Here's how the part is built. I have some questions about the finished solid (model axes, mm). Coordinates: 2 decimals unless noted, no trailing zeros. Answer as a JSON object with one key per item and string values. Group by question number.
Q1. I'm going to push flat-ended pins straight in: pin 1 (1.5 mm diameter, centred on x = -8.5, y = -60.5, fed in from -Z); pin 2 (1 mm diameter, centred on x = 0.13, y = 0, fed in from +Z). Where does each tip first touch, or does it pass through?
Q2. I want a section at A-A on z = 1.25. Count the separate pieces of the cut face and the enclosed holes in it, then the cut area to 3 significant figures.
Q3. I need wall thicknesses on line 1 (Y direction, x = -27, z = 0.7); line 2 (Y direction, x = 0, z = 1.6); line 3 (X direction, y = 18.5, z = 1.15). Which ranges of each line are inside material? Lowest first, please.
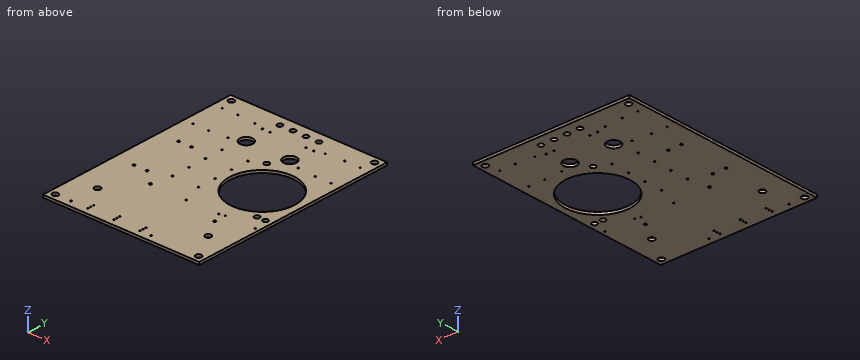
```python
from build123d import *

# Parameters (mm, degrees)
SKETCH_1_W          = 120
SKETCH_1_H          = 160
SKETCH_1_R          = 2.25
SKETCH_1_R_2        = 25
EXTRUDE_1_DEPTH     = 2
SKETCH_2_R          = 2.25
SKETCH_2_R_2        = 0.6
SKETCH_2_R_3        = 0.5
SKETCH_2_R_4        = 2
CUT_EXTRUDE_1_DEPTH = 2
SKETCH_3_R          = 5
SKETCH_3_R_2        = 0.6
SKETCH_3_R_3        = 1
CUT_EXTRUDE_2_DEPTH = 2
SKETCH_4_R          = 0.9
SKETCH_4_R_2        = 0.6
CUT_EXTRUDE_3_DEPTH = 2
SKETCH_5_R          = 0.5
CUT_EXTRUDE_4_DEPTH = 2


with BuildPart() as part:
    # Эскиз1 → Вытянуть1 (new body)
    with BuildSketch(Plane.XY):
        Rectangle(SKETCH_1_W, SKETCH_1_H)
        with Locations((-55, -75)):
            Circle(SKETCH_1_R, mode=Mode.SUBTRACT)
        with Locations((55, -75)):
            Circle(SKETCH_1_R, mode=Mode.SUBTRACT)
        with Locations((55, 75)):
            Circle(SKETCH_1_R, mode=Mode.SUBTRACT)
        with Locations((-55, 75)):
            Circle(SKETCH_1_R, mode=Mode.SUBTRACT)
        with Locations((30, 7)):
            Circle(SKETCH_1_R_2, mode=Mode.SUBTRACT)
    extrude(amount=EXTRUDE_1_DEPTH)

    # Эскиз2 → Вырез-Вытянуть1 (cut)
    with BuildSketch(Plane.XY.offset(2)):
        with Locations((-42, -53.5)):
            Circle(SKETCH_2_R)
        with Locations((43, -53.5)):
            Circle(SKETCH_2_R)
        with Locations((-43, -75)):
            Circle(SKETCH_2_R_2)
        with Locations((18.5, -75)):
            Circle(SKETCH_2_R_2)
        with Locations((-30, -70)):
            Circle(SKETCH_2_R_3)
        with Locations((-30, -72.5)):
            Circle(SKETCH_2_R_3)
        with Locations((-30, -75)):
            Circle(SKETCH_2_R_3)
        with Locations((-10, -70)):
            Circle(SKETCH_2_R_3)
        with Locations((-10, -72.5)):
            Circle(SKETCH_2_R_3)
        with Locations((-10, -75)):
            Circle(SKETCH_2_R_3)
        with Locations((10, -70)):
            Circle(SKETCH_2_R_3)
        with Locations((10, -72.5)):
            Circle(SKETCH_2_R_3)
        with Locations((10, -75)):
            Circle(SKETCH_2_R_3)
        with Locations((-15, 72)):
            Circle(SKETCH_2_R_4)
        with Locations((-5, 72)):
            Circle(SKETCH_2_R_4)
        with Locations((5, 72)):
            Circle(SKETCH_2_R_4)
        with Locations((15, 72)):
            Circle(SKETCH_2_R_4)
        with Locations((10, 33)):
            Circle(SKETCH_2_R_4)
        with Locations((55, -18)):
            Circle(SKETCH_2_R_4)
        with Locations((48.5, -18)):
            Circle(SKETCH_2_R_4)
    extrude(amount=-CUT_EXTRUDE_1_DEPTH, mode=Mode.SUBTRACT)

    # Эскиз3 → Вырез-Вытянуть2 (cut)
    with BuildSketch(Plane.XY.offset(2)):
        with Locations((-16.5, 45)):
            Circle(SKETCH_3_R)
        with Locations((17, 45)):
            Circle(SKETCH_3_R)
        with Locations((-19.5, 62)):
            Circle(SKETCH_3_R_2)
        with Locations((-13.5, 62)):
            Circle(SKETCH_3_R_2)
        with Locations((14, 62)):
            Circle(SKETCH_3_R_2)
        with Locations((20, 62)):
            Circle(SKETCH_3_R_2)
        with Locations((34, -38)):
            Circle(SKETCH_3_R_3)
        with Locations((-23, -29.5)):
            Circle(SKETCH_3_R_3)
    extrude(amount=-CUT_EXTRUDE_2_DEPTH, mode=Mode.SUBTRACT)

    # Эскиз4 → Вырез-Вытянуть3 (cut)
    with BuildSketch(Plane.XY.offset(2)):
        with Locations((-45, 19)):
            Circle(SKETCH_4_R)
        with Locations((-35, 19)):
            Circle(SKETCH_4_R)
        with Locations((-35, -19)):
            Circle(SKETCH_4_R)
        with Locations((-45, -19)):
            Circle(SKETCH_4_R)
        with Locations((-20, -14)):
            Circle(SKETCH_4_R_2)
        with Locations((0, -14)):
            Circle(SKETCH_4_R_2)
        with Locations((-19.873847439, 0)):
            Circle(SKETCH_4_R_2)
        with Locations((0.126152561, 0)):
            Circle(SKETCH_4_R_2)
        with Locations((-20, 14)):
            Circle(SKETCH_4_R_2)
        with Locations((0, 14)):
            Circle(SKETCH_4_R_2)
        with Locations((-20, 28)):
            Circle(SKETCH_4_R_2)
        with Locations((0, 28)):
            Circle(SKETCH_4_R_2)
    extrude(amount=-CUT_EXTRUDE_3_DEPTH, mode=Mode.SUBTRACT)

    # Эскиз5 → Вырез-Вытянуть4 (cut)
    with BuildSketch(Plane.XY.offset(2)):
        with Locations((-53, 40)):
            Circle(SKETCH_5_R)
        with Locations((-53, 65)):
            Circle(SKETCH_5_R)
        with Locations((-41, 40)):
            Circle(SKETCH_5_R)
        with Locations((-41, 65)):
            Circle(SKETCH_5_R)
        with Locations((41, 40)):
            Circle(SKETCH_5_R)
        with Locations((41, 65)):
            Circle(SKETCH_5_R)
        with Locations((53, 40)):
            Circle(SKETCH_5_R)
        with Locations((53, 65)):
            Circle(SKETCH_5_R)
        with Locations((-27, 41)):
            Circle(SKETCH_5_R)
        with Locations((-27, 64)):
            Circle(SKETCH_5_R)
        with Locations((27, 41)):
            Circle(SKETCH_5_R)
        with Locations((27, 64)):
            Circle(SKETCH_5_R)
        with Locations((34, -29)):
            Circle(SKETCH_5_R)
        with Locations((57, -29)):
            Circle(SKETCH_5_R)
        with Locations((5, -30)):
            Circle(SKETCH_5_R)
        with Locations((30, -30)):
            Circle(SKETCH_5_R)
    extrude(amount=-CUT_EXTRUDE_4_DEPTH, mode=Mode.SUBTRACT)


solid = part.part
```
Result set:
{
 "1": {"pin 1": "stops at z = 0", "pin 2": "passes through"},
 "2": {"separate pieces": "1", "enclosed holes": "61", "area": "16,800 mm²"},
 "3": {"line 1": "y = -80 to 40.5, 41.5 to 63.5, 64.5 to 80", "line 2": "y = -80 to -14.6, -13.4 to -0.59, 0.59 to 13.4, 14.6 to 27.4, 28.6 to 80", "line 3": "x = -60 to -45.75, -44.25 to -35.75, -34.25 to 7.8, 52.2 to 60"}
}
